Source: CAD feature listing. Evaluate the final solid. Frame: model axes, mm. A direction names the side the tool comes from. Coordinates: 2 decimals unless noted, no trailing zeros. Order: outer loops, then holes, each group sorted by start corner. A loop starts at its lowest first (then second) coordinate and runs counter-clockwise, first axis right, second up. Notation, with made-up numbers: (-22, -27) - (24, -27) arc R21 ccw to (24, -16) - close; hole circle Ø10 at (-40, -31.5). An arc over 180 degrees is marked (long way). One line per question, with ' | ' between items. Start each with the question number.
(1) Contact query for flat-ended pins moving along their axis: P1, Ø2, axis at x = 109, y = -10, coming from the -Z side; P2, Ø1, axis at x = 105, z = 5.5, coming from the +Y side; P3, Ø10, axis at x = 106.5, y = 12, coming from the +Z side. Output: stop coordinate, or through.
(2) Line query: line 1 along X through (y, z) = (-40.5, -10.5); line 2 along X through (y, z) = (4, 30); line 3 along Z through (x, y) = (157, -12). Output: solid intervals per line, ascending.
(3) Draft query along X for faces 1 (the flat face through (107.474, 19.328, 32.213)), 2 (the flat face through (214, -31, 9)), 3 (the flat face through (218, -33, 17)). Return one class per face: +X half, -X half, draft (parallel to the pull), parting line (faces both ways), or undercut.
(4) Section C-C (z = 45). Return the cut outline in (x, y).
(5) Section B-B (z = -35.5). Return the cut outline in (x, y).
(6) Section D-D (y = 26). Return the cut outline in (x, z).
(7) Access query for faces 4 (the cylindrical face through (207.986, -25.703, -1.972)), 5 (the flat face through (108, 14, 30)), 6 (the flat face through (24, -13, -4)), 7 (the flat face through (4, -29, 4)). Directions: +Z, -Z, +X, -X, +Y, -Y. A direction counts if a zero-diameter tool reaches every point of the face in a straight line with its end or side. Return the directions, or none.
(8) Section A-A (y = -49.5). Return the cut outline in (x, z), then the cut area to 4 significant figures.
from build123d import *

# Parameters (mm, degrees)
SALIENTE_EXTRUIR1_DEPTH = 218
CROQUIS4_W              = 40.00000000000003
CROQUIS4_H              = 96.00000000000001
CORTAR_EXTRUIR1_DEPTH   = 60
CORTAR_EXTRUIR2_DEPTH   = 4
REDONDEO1_R             = 20


with BuildPart() as part:
    # Croquis2 → Saliente-Extruir1 (new body)
    with BuildSketch(Plane(origin=(0, 0, 0), x_dir=(0, 0, -1), z_dir=(1, 0, 0))):
        Polygon((-60.000000000000014, 35.99999999999998), (-59.99999999999997, -60), (100, -59.99999999999999), align=None)
    extrude(amount=SALIENTE_EXTRUIR1_DEPTH)

    # Croquis3 → Cortar-Recubrir1 section 0
    with BuildSketch(Plane.XY.offset(60)):
        with BuildLine():
            Line((4, 32), (214, 32))
            Line((214, 32), (214, -59.99999999999997))
            Line((214, -59.99999999999997), (4.0000000000000115, -59.99999999999997))
            Line((4.0000000000000115, -59.99999999999997), (4, 32))
        make_face()
    # Croquis3D3 → Cortar-Recubrir1 section 1
    with BuildSketch(Plane(origin=(4, -3.9999999999999964, 0), x_dir=(0.9662349396012463, -0.25766265056033233, 0), z_dir=(0, 0, 1))):
        with BuildLine():
            Line((0, 0), (202.9093373162617, 54.10915661766981))
            Line((202.9093373162617, 54.10915661766981), (217.33844574764032, 0))
            Line((217.33844574764032, 0), (14.42910843137861, -54.1091566176698))
            Line((14.42910843137861, -54.1091566176698), (0, 0))
        make_face()
    loft(mode=Mode.SUBTRACT)

    # Croquis4 → Cortar-Extruir1 (cut)
    with BuildSketch(Plane.XZ.offset(60)):
        Polygon((3.999999999999988, -4), (43.99999999999999, -4), (44.00000000000001, -100), (4, -100), align=None)
        Polygon((46.499999999999986, -4), (86.49999999999999, -4), (86.5, -100), (46.5, -100), align=None)
        Polygon((88.99999999999999, -3.9999999999999973), (128.99999999999997, -3.9999999999999973), (128.99999999999997, -100), (89, -100), align=None)
        with Locations((151.5, -52.00000000000001)):
            Rectangle(CROQUIS4_W, CROQUIS4_H)
        with Locations((194, -52.00000000000001)):
            Rectangle(CROQUIS4_W, CROQUIS4_H)
    extrude(amount=-CORTAR_EXTRUIR1_DEPTH, mode=Mode.SUBTRACT)

    # Croquis5 → Cortar-Extruir2 (cut)
    with BuildSketch(Plane(origin=(0, 1.7e-16, -4), x_dir=(-1, 0, 0), z_dir=(0, 4e-17, -1))):
        Polygon((-194, -60), (-174.00000000000003, -60.00000000000001), (-174.00000000000003, -19.99999999999999), (-214, -19.999999999999996), (-214, -60), align=None)
        Polygon((-151.49999999999997, -60), (-131.49999999999997, -60), (-131.49999999999997, -19.99999999999999), (-171.5, -19.999999999999996), (-171.49999999999997, -60), align=None)
        Polygon((-108.99999999999999, -60), (-88.99999999999999, -60), (-88.99999999999999, -19.999999999999996), (-128.99999999999997, -20), (-128.99999999999997, -60), align=None)
        Polygon((-66.49999999999997, -60), (-46.49999999999997, -60), (-46.49999999999997, -19.999999999999996), (-86.5, -19.999999999999996), (-86.49999999999999, -60), align=None)
        Polygon((-23.99999999999999, -60), (-3.99999999999999, -60), (-3.99999999999999, -19.99999999999999), (-43.99999999999999, -19.999999999999996), (-43.99999999999999, -60), align=None)
    extrude(amount=-CORTAR_EXTRUIR2_DEPTH, mode=Mode.SUBTRACT)

    # Redondeo1
    redondeo1_edges = [part.edges().sort_by_distance(p)[0] for p in [
        (3.99999999999999, -19.99999999999999, -2.000000000000001),
        (43.99999999999999, -19.999999999999996, -2.000000000000001),
        (46.49999999999997, -19.999999999999996, -2.000000000000001),
        (86.5, -19.999999999999996, -2.000000000000001),
        (88.99999999999999, -19.999999999999996, -2.000000000000001),
        (128.99999999999997, -20, -2.000000000000001),
        (131.49999999999997, -19.99999999999999, -2.000000000000001),
        (171.5, -19.999999999999996, -2.000000000000001),
        (174.00000000000003, -19.99999999999999, -2.000000000000001),
        (214, -19.999999999999996, -2.000000000000001),
    ]]
    fillet(redondeo1_edges, radius=REDONDEO1_R - 0.0001)  # a hair under: the kernel refuses the full size


solid = part.part
Response values:
1) P1: stops at z = -4 | P2: stops at y = 3.6 | P3: stops at z = 35
2) line 1: x = 0 to 4, 44 to 46.5, 86.5 to 89, 129 to 131.5, 171.5 to 174, 214 to 218 | line 2: x = 0 to 4, 214 to 218 | line 3: z = -4 to 0
3) face 1: draft | face 2: undercut | face 3: +X half
4) outline: (0, -60) - (4, -60) - (4, 23) - (214, 23) - (214, -60) - (218, -60) - (218, 27) - (0, 27) - close
5) outline: (0, -60) - (4, -60) - (4, -21.3) - (0, -21.3) - close; (44, -60) - (46.5, -60) - (46.5, -21.3) - (44, -21.3) - close; (86.5, -60) - (89, -60) - (89, -21.3) - (86.5, -21.3) - close; (129, -60) - (131.5, -60) - (131.5, -21.3) - (129, -21.3) - close; (171.5, -60) - (174, -60) - (174, -21.3) - (171.5, -21.3) - close; (214, -60) - (218, -60) - (218, -21.3) - (214, -21.3) - close
6) outline: (0, 43.33) - (218, 43.33) - (218, 60) - (214, 60) - (214, 50) - (4, 50) - (4, 60) - (0, 60) - close
7) face 4: +Z, -Z, -Y | face 5: +Z, -Y | face 6: -Z, +Y, -Y | face 7: -Y
8) outline: (0, -82.5) - (4, -82.5) - (4, 60) - (0, 60) - close; (44, -82.5) - (46.5, -82.5) - (46.5, 0) - (44, 0) - close; (86.5, -82.5) - (89, -82.5) - (89, 0) - (86.5, 0) - close; (129, -82.5) - (131.5, -82.5) - (131.5, 0) - (129, 0) - close; (171.5, -82.5) - (174, -82.5) - (174, 0) - (171.5, 0) - close; (214, -82.5) - (218, -82.5) - (218, 60) - (214, 60) - close | area: 1,965 mm²
